Autodesk Inventor part; units mm, degrees
ref_plane "YZ Plane" through (0, 0, 0) normal (1, 0, 0) x (0, 1, 0)
ref_plane "XZ Plane" through (0, 0, 0) normal (0, 1, 0) x (-1, 0, 0)
ref_plane "XY Plane" through (0, 0, 0) normal (0, 0, 1) x (1, 0, 0)
sketch "Sketch1" plane through (0, 0, 0) normal (0, 0, 1) x (1, 0, 0)
  arc A0 (0, 0) -> (39.7002, -68.7324) centre (79.375, 0.0157) ccw
  line L0 (39.7002, -68.7324) -> (139.7567, -51.0897)
  line L1 (39.7002, -68.7324) -> (141.3002, -68.7324) construction
  arc A1 (136.4379, -51.6749) -> (205.7416, -92.3565) centre (205.743, -12.9815) ccw
  arc A2 (139.7567, -51.0897) -> (205.7416, -89.1815) centre (205.743, -12.9815) ccw
  line L2 (205.7416, -89.1815) -> (205.7416, -92.3565)
  line L3 (0, 0) -> (205.7416, 0)
  line L4 (205.7416, 0) -> (205.7416, -89.1815)
  dimension "d0" = 79.375
  dimension "d1" = 68.7324
  dimension "d2" = 39.7002
  dimension "d3" = 101.6
  dimension "d4" = 10
  dimension "d5" = 79.375
  dimension "d6" = 76.2
  dimension "d7" = 3.175
  dimension "d9" = 0
  dimension "d10" = 0
  dimension "d11" = 48.9712
extrude "Extrusion1" add sketch "Sketch1" along normal blind 3.175
sketch "Sketch2" plane through (0, 0, 3.175) normal (0, 0, 1) x (1, 0, 0)
  line L0 (205.7416, -92.3565) -> (205.7416, 0)
  line L1 (205.7416, -3.4565) -> (218.4416, -3.4565)
  line L2 (218.4416, -3.4565) -> (218.4416, -16.1565)
  line L3 (218.4416, -16.1565) -> (205.7416, -16.1565)
  line L4 (205.7416, -16.1565) -> (205.7416, -3.4565)
  circle A0 centre (212.0916, -9.8065) radius 3.175
  point P0 (0, 0)
  dimension "d14" = 12.7
  dimension "d15" = 12.7
  dimension "d16" = 92.3565
  dimension "d17" = 6.35
  dimension "d18" = 82.55
  dimension "d19" = 6.35
extrude "Extrusion2" add sketch "Sketch2" against normal blind 3.175
sketch "Sketch3" plane through (0, 0, 3.175) normal (0, 0, 1) x (1, 0, 0)
  circle A0 centre (212.0916, -9.8065) radius 3.175
  arc A1 (0, 0) -> (39.7002, -68.7324) centre (79.375, 0.0157) ccw
  line L0 (39.7002, -68.7324) -> (136.4379, -51.6749)
  arc A2 (136.4379, -51.6749) -> (205.7416, -92.3565) centre (205.743, -12.9815) ccw
  line L1 (205.7416, -92.3565) -> (205.7416, -16.1565)
  line L2 (218.4416, -16.1565) -> (205.7416, -16.1565)
  line L3 (218.4416, -3.4565) -> (218.4416, -16.1565)
  line L4 (205.7416, -3.4565) -> (218.4416, -3.4565)
  line L5 (205.7416, -3.4565) -> (205.7416, 0)
  line L6 (205.7416, 0) -> (0, 0)
  line L7 (205.7416, 0) -> (0, 0)
  line L8 (142.7882, 0) -> (123.7382, 0)
  line L9 (123.7382, 0) -> (123.7382, 37.2251)
  line L10 (123.7382, 37.2251) -> (142.7882, 37.2251)
  line L11 (142.7882, 37.2251) -> (142.7882, 0)
  dimension "d22" = 19.05
  dimension "d23" = 88.9
  dimension "d25" = 47.0315
  dimension "d26" = 69.3034
extrude "Extrusion3" add sketch "Sketch3" against normal blind 3.175 contours L9 L10 L11 L6
sketch "Sketch4" plane through (0, 0, 3.175) normal (0, 0, 1) x (1, 0, 0)
  circle A0 centre (212.0916, -9.8065) radius 3.175
  arc A1 (0, 0) -> (39.7002, -68.7324) centre (79.375, 0.0157) ccw
  line L0 (39.7002, -68.7324) -> (136.4379, -51.6749)
  arc A2 (136.4379, -51.6749) -> (205.7416, -92.3565) centre (205.743, -12.9815) ccw
  line L1 (205.7416, -92.3565) -> (205.7416, -16.1565)
  line L2 (218.4416, -16.1565) -> (205.7416, -16.1565)
  line L3 (218.4416, -3.4565) -> (218.4416, -16.1565)
  line L4 (205.7416, -3.4565) -> (218.4416, -3.4565)
  line L5 (205.7416, -3.4565) -> (205.7416, 0)
  line L6 (205.7416, 0) -> (142.7882, 0)
  line L7 (142.7882, 0) -> (142.7882, 37.2251)
  line L8 (142.7882, 37.2251) -> (123.7382, 37.2251)
  line L9 (123.7382, 37.2251) -> (123.7382, 0)
  line L10 (123.7382, 0) -> (0, 0)
  point P0 (133.2632, 30.8751)
  point P1 (133.2632, 11.3171)
  point P2 (183.2626, -9.8065)
  point P3 (163.7046, -9.8065)
  dimension "d29" = 9.525
  dimension "d30" = 6.35
  dimension "d31" = 19.558
  dimension "d32" = 9.525
  dimension "d33" = 28.829
  dimension "d35" = 0
  dimension "d36" = 0
  dimension "d44" = 19.558
hole "Hole1" at (133.2632, 30.8751, 3.175) at (133.2632, 11.3171, 3.175) at (183.2626, -9.8065, 3.175) at (163.7046, -9.8065, 3.175) direction (0, 0, -1) diameter 3.81 end through all
equation "\"d19\" = 0.5 * d15"
properties part number "CollectionCasing"
Geometry check sheet. Reference: the model listing, model coordinates, mm. A direction names the side the tool comes from. Round coordinates to 2 decimals unless told otherwise and drop trailing zeros. Loops run counter-clockwise (first coordinate to the right, second up) from the corner with the lowest first, then second, coordinate; pieces in that order, holes last.
Item 1: Mould release check, pull along X, two halves, no side actions. Record for faces 3 (the flat face through (132, -41, 0)), 4 (the cylindrical face through (10.935, -40.188, 1.565)), 5 (the flat face through (87.392, -60.323, 1.565)): pulls with the +X half, pulls with the -X half, needs draft (parallel to the pull), parting line crosses it, or undercut.
Item 2: Access from +Z, -Z, +X, -X, +Y, -Y to the whole of each face (thin tool, end or side, straight path). Record for faces 1 (the cylindrical face through (215.024, -11.023, 1.61)), 2 (the cylindrical face through (166.07, -81.73, 1.57)).
Item 3: Cross-section at A-A on y = -64. Record the boundary of the cut face in (x, z) (3 decimals).
Item 4: Cross-section at D-D on x = 53. Record the boundary of the cut face in (y, z) (3 decimals).
Item 5: Cross-section at B-B on z = 1.6. Count the separate pieces of the cut face and the enclosed holes in it, then the cut area to 3 significant figures.
Item 6: Thickness scan on line 1 (X direction, y = -10.5, z = 0.3); line 2 (X direction, y = 19.5, z = 2.2); line 3 (X direction, y = -8.5, z = 2). Record the ranges inside material, lowest first.
Item 7: Gauge pin test, flat ends, axial feed: pin 1 (1.6 mm diameter, centred on y = -51, z = 2, fed in from +X); pin 2 (2.5 mm diameter, centred on x = 163.7, y = -9.81, fed in from -Z); pin 3 (1 mm diameter, centred on y = 12, z = 1.5, fed in from -X); pin 4 (1.6 mm diameter, centred on y = 15, z = 1, fed in from +X). Record the tip position at first contact, or that the pin passes through.
Item 8: Cross-section at C-C on y = 26.5. Record the boundary of the cut face in (x, z) (3 decimals), then the cut area to 3 significant figures.
Answer sheet:
1. face 3: needs draft
1. face 4: pulls with the -X half
1. face 5: undercut
2. face 1: +Z, -Z
2. face 2: +Z, -Z, -Y
3. outline: (32.445, 0) - (66.539, 0) - (66.539, 3.175) - (32.445, 3.175) - close; (144.936, 0) - (205.742, 0) - (205.742, 3.175) - (144.936, 3.175) - close
4. outline: (-66.387, 0) - (0, 0) - (0, 3.175) - (-66.387, 3.175) - close
5. separate pieces: 1
5. enclosed holes: 5
5. area: 14,100 mm2
6. line 1: x = 0.7 to 161.93, 165.48 to 181.49, 185.04 to 208.99, 215.19 to 218.44
6. line 2: x = 123.74 to 142.79
6. line 3: x = 0.46 to 162.32, 165.09 to 181.88, 184.65 to 209.2, 214.99 to 218.44
7. pin 1: stops at x = 205.74
7. pin 2: passes through
7. pin 3: stops at x = 123.74
7. pin 4: stops at x = 142.79
8. outline: (123.738, 0) - (142.788, 0) - (142.788, 3.175) - (123.738, 3.175) - close
8. area: 60.5 mm2
